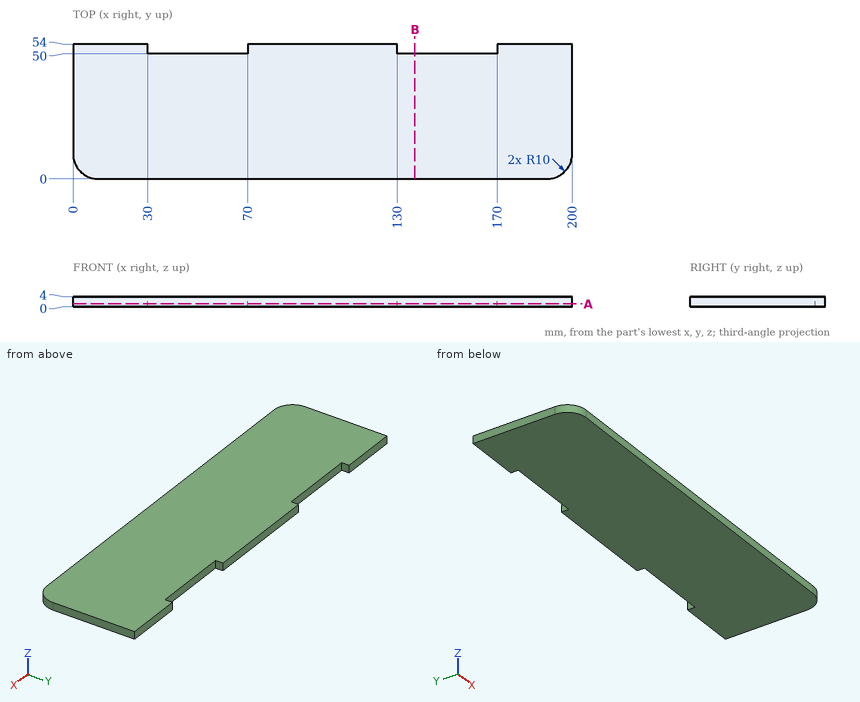
Input: dimensioned drawing with shaded views. Units: mm. Origin: part minimum x, y, z. Coordinates: 2 decimals unless noted, no trailing zeros. Write each loop counter-clockwise with the first axis right and the second up, starting at its lowest first coordinate (ties: lowest second). Pieces come first, ordered by that corner, then holes. Notation, with made-up numbers: M 24.5,79 L 61.5,79 A32 ccw 61.5,111 Z; hole C -33,77 d11. An arc over 180 degrees is marked long. Answer as a JSON object with one key per item and string values. Group by question number.
(1) Section A-A on z = 1.15. Output: boundary loops of the cut face in (x, y).
(2) Ray query, line 1 along Y through (x, z) = (39, 3.45); line 2 along X through (y, z) = (4, 2.9); line 3 along X through (y, z) = (4.5, 3.5). Return the intervals inside material, ascending. Write a range as [from, to].
(3) Section B-B on x = 137. Output: boundary loops of the cut face in (y, z), plus the area to 3 significant figures.
(4) Contact query for a flat-ended pin moving along its axis: P1, Ø1.2, axis at x = 141, z = 1, coming from the +Y side. Output: stop coordinate, or through.
Result set:
{
 "1": {"outline": "M 0,10 A10 ccw 10,0 L 190,0 A10 ccw 200,10 L 200,54 L 170,54 L 170,50 L 130,50 L 130,54 L 70,54 L 70,50 L 30,50 L 30,54 L 0,54 Z"},
 "2": {"line 1": "y = [0, 50]", "line 2": "x = [2, 198]", "line 3": "x = [1.65, 198.35]"},
 "3": {"outline": "M 0,0 L 50,0 L 50,4 L 0,4 Z", "area": "200 mm2"},
 "4": {"P1": "stops at y = 50"}
}
